For this review, take the finished solid that the model builds, in its own axes (mm). Face numbers are marked on the shaded views. A direction names the side the tool comes from. Give positions to 0.01 mm unless a question says otherwise; leave off trailing zeros. Order: outer loops, then holes, each group sorted by start corner. A loop starts at its lowest first (then second) coordinate and runs counter-clockwise, first axis right, second up.
Item 1: Consider section D-D (y = -13.5). Give the boundary of the cut face in (x, z), plus the area to 3 significant figures.
Item 2: Consider section B-B (z = -4.25). Give the boundary of the cut face in (x, y).
Item 3: For probe 1 along Y at (x, z) = (6.5, 15); probe 2 along Y at (x, z) = (0.5, 11.75); probe 3 along Z at (x, y) = (-0.25, -17), list the stretches that pass through material, from the lowest coordinate up.
Item 4: For P1, Ø3, axis at x = 5.5, z = 15.5, coming from the -Y side; P2, Ø10, axis at y = -18, z = 3, coming from the +X side; P3, Ø5, axis at x = 3.5, y = -18.5, coming from the -Z side; P4, Ø12.5, axis at x = 6.5, z = 2.5, coming from the -Y side, all flat-tipped, find the tip position at first contact; note any pin that passes through.
Item 5: Consider section A-A (x = 0). Give the boundary of the cut face in (y, z), plus the area to 3 significant figures.
Item 6: Machinability: for the marked faces 1 and 2, which of the approach directions +Z, -Z, +X, -X, +Y, -Y give a long, thin tool a straight path to every point of the face, cutting with its end or side? Answer none if there is none.
Item 7: Consider section C-C (x = 10.5). Give the boundary of the cut face in (y, z), plus the area to 3 significant figures.
```python
from build123d import *

# Parameters (mm, degrees)
F0_R     = 7.62
F1_DEPTH = 25.4
F2_R     = 2.54
F4_DEPTH = 6.35


with BuildPart() as f1:
    # F0 (on Front) → F1 (new body)
    with BuildSketch(Plane.XZ):
        with Locations((0, 6.581996)):
            Circle(F0_R)
    extrude(amount=F1_DEPTH)

    # F2
    f2_edges = [f1.edges().sort_by_distance(p)[0] for p in [
        (-7.62, -25.4, 6.581996),
    ]]
    fillet(f2_edges, radius=F2_R)

    # F3 (on Front) → F4 (join)
    with BuildSketch(Plane.XZ):
        Polygon((-12.7, 19.281996), (-12.7, 15.119903), (-12.7, -6.118004), (12.7, -6.118004), (12.7, 19.281996), align=None)
    extrude(amount=-F4_DEPTH)


solid = f1.part
```
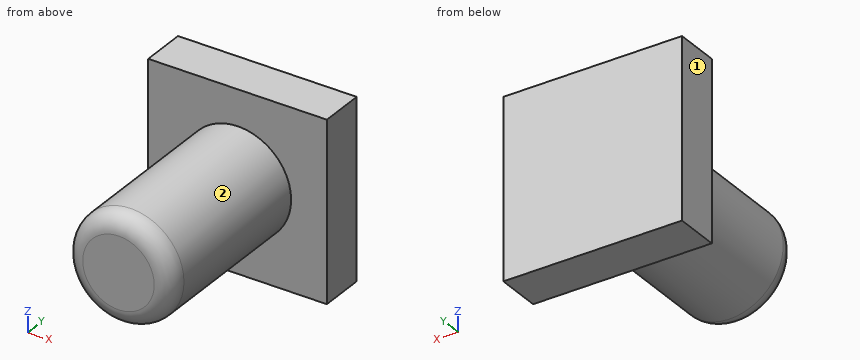
Resolved:
1. outline: circle Ø15.24 at (0, 6.58)
1. area: 182 mm2
2. outline: (-12.7, 0) - (12.7, 0) - (12.7, 6.35) - (-12.7, 6.35) - close
3. probe 1: y = 0 to 6.35
3. probe 2: y = -25.4 to 6.35
3. probe 3: z = -1.03 to 14.2
4. P1: stops at y = 0
4. P2: stops at x = 7.62
4. P3: stops at z = -0.97
4. P4: stops at y = -25.4
5. outline: (-25.4, 1.5) arc R2.54 ccw to (-22.86, -1.04) - (0, -1.04) - (0, -6.12) - (6.35, -6.12) - (6.35, 19.28) - (0, 19.28) - (0, 14.2) - (-22.86, 14.2) arc R2.54 ccw to (-25.4, 11.66) - close
5. area: 546 mm2
6. face 1: +Z, -Z, -X, +Y, -Y
6. face 2: -Y
7. outline: (0, -6.12) - (6.35, -6.12) - (6.35, 19.28) - (0, 19.28) - close
7. area: 161 mm2
